from build123d import *

# Parameters (mm, degrees)
F0_R     = 4.5
F0_R_2   = 2.9
F0_R_3   = 2.1
F1_DEPTH = 8
F2_DEPTH = 8.001
F3_DEPTH = 5
F4_SIZE  = 0.25


with BuildPart() as f1:
    # F0 (on Top) → F1 (new body)
    with BuildSketch(Plane.XY):
        Circle(F0_R)
        Circle(F0_R_2, mode=Mode.SUBTRACT)
        Circle(F0_R_2)
        Circle(F0_R_3, mode=Mode.SUBTRACT)
        Circle(F0_R_3)
    extrude(amount=F1_DEPTH)

    # F0 (on Top) → F2 (cut, through all)
    with BuildSketch(Plane.XY):
        Circle(F0_R_3)
    extrude(amount=F2_DEPTH, mode=Mode.SUBTRACT)

    # F0 (on Top) → F3 (cut)
    with BuildSketch(Plane.XY):
        Circle(F0_R_2)
        Circle(F0_R_3, mode=Mode.SUBTRACT)
    extrude(amount=F3_DEPTH, mode=Mode.SUBTRACT)

    # F4
    f4_edges = [f1.edges().sort_by_distance(p)[0] for p in [
        (-2.1, 0, 5),
        (-2.9, 0, 0),
        (-4.5, 0, 0),
    ]]
    chamfer(f4_edges, length=F4_SIZE)


solid = f1.part
The listing builds one solid part. Answer for the finished solid, in the listing's coordinates (mm). Coordinates: 2 decimals unless noted, no trailing zeros. Loops run counter-clockwise (first coordinate to the right, second up) from the corner with the lowest first, then second, coordinate; pieces in that order, holes last. Notation, with made-up numbers: (66, -34) -> (93, -34) arc R22 cw to (93, -19) -> close; hole circle Ø8 at (88, 44.5). An arc over 180 degrees is marked (long way). Write item = value, one per line. Start each with the question number.
1) The mould has two halves that part along Y. Classify faces 1 (the face through (-2.9, 0.1, 2.6)), 2 (the face through (-0.59, 4.46, 4.07)), 3 (the face through (-2.1, -0.9, 8)): released by +Y, released by -Y, zero draft, split by the parting line, or undercut.
2) A cutting plane is placed at C-C (z = 6.5). Give the vertices of the cut face in (x, y).
3) Straight lines are drawn through the part: line 1 (Y direction, x = 0, z = 6.8); line 2 (Y direction, x = 0, z = 3.65); line 3 (Z direction, x = 0.25, y = -2.75). For each, find the intervals that lie inside material, in ascending order. Write a range as from..to.
4) A cutting plane is placed at A-A (x = 0). Give the vertices of the cut face in (y, z).
5) A cutting plane is placed at D-D (z = 1). Give the vertices of the cut face in (x, y), then the cut area to 3 significant figures.
6) Given pin 1 Ø3 at (x, y) = (-1, -0.5) entering from -Z; pin 2 Ø2 at (y, z) = (1.5, 6.5) entering from -X; pin 3 Ø2 at (y, z) = (-1.5, 4.5) entering from +X, each flat-ended and moving along its own axis, determine where each tip first touches the part or whether it passes through.
Responses:
q1.face_1 = undercut
q1.face_2 = split by the parting line
q1.face_3 = zero draft
q2.outline = circle Ø9 at (0, 0); hole circle Ø4.2 at (0, 0)
q3.line_1 = -4.5..-2.1, 2.1..4.5
q3.line_2 = -4.5..-2.9, 2.9..4.5
q3.line_3 = 5..8
q4.outline = (-4.5, 0.25) -> (-4.25, 0) -> (-3.15, 0) -> (-2.9, 0.25) -> (-2.9, 5) -> (-2.35, 5) -> (-2.1, 5.25) -> (-2.1, 8) -> (-4.5, 8) -> close; (2.1, 5.25) -> (2.35, 5) -> (2.9, 5) -> (2.9, 0.25) -> (3.15, 0) -> (4.25, 0) -> (4.5, 0.25) -> (4.5, 8) -> (2.1, 8) -> close
q5.outline = circle Ø9 at (0, 0); hole circle Ø5.8 at (0, 0)
q5.area = 37.2 mm²
q6.pin_1 = 5
q6.pin_2 = -4.47
q6.pin_3 = 4.47
